Autodesk Inventor part; units mm, degrees
ref_plane "YZ Plane" through (0, 0, 0) normal (1, 0, 0) x (0, 1, 0)
ref_plane "XZ Plane" through (0, 0, 0) normal (0, 1, 0) x (-1, 0, 0)
ref_plane "XY Plane" through (0, 0, 0) normal (0, 0, 1) x (1, 0, 0)
sketch "Skizze1" plane through (0, 0, 0) normal (0, 1, 0) x (-1, 0, 0)
  circle A0 centre (0, 0) radius 12.25
  dimension "d0" = 24.5
extrude "Extrusion1" add sketch "Skizze1" along normal blind 9.5
sketch "Skizze2" plane through (0, 9.5, 0) normal (0, 1, 0) x (1, 0, 0)
  circle A0 centre (0, 0) radius 12.75
  dimension "d3" = 25.5
extrude "Extrusion2" add sketch "Skizze2" along normal blind 1.5
sketch "Skizze3" plane through (0, 0, 0) normal (0, -1, 0) x (1, 0, 0)
  circle A0 centre (0, 0) radius 12.25
hole "Bohrung1" at (0, 0, 0) direction (0, 1, 0) diameter 21 depth 9.5
properties part number "17"
Geometry: final body of the model. Coordinates: model frame, mm. Round coordinates to 2 decimals unless told otherwise and drop trailing zeros. Order: outer loops, then holes, each group sorted by start corner. A loop starts at its lowest first (then second) coordinate and runs counter-clockwise, first axis right, second up. Notation, with made-up numbers: (-13.5, 74) -> (27.5, 74) arc R24 ccw to (27.5, 94) -> close; hole circle Ø9 at (26, 81). An arc over 180 degrees is marked (long way). Put each result on its own line as item: value. Start each with the question number.
Q1. Section A-A on x = 0. Return the cut outline in (y, z).
Q2. Pull-direction query (Z, two-part tool) for faces 1 (the flat face through (0, 9.5, 0)), 2 (the cylindrical face through (-6.586, 4.684, -10.329)), 3 (the cylindrical face through (-3.2, 4.8, -10)), 4 (the flat face through (0, 11, 0)); classes: +Z half, -Z half, draft (parallel to the pull), parting line (faces both ways), or undercut.
Q3. Section D-D on z = 11.25. Return the cut outline in (x, y), and give its area (3 significant figures).
Q4. First-contact query: pin 1 (1 mm diameter, centred on x = 8, y = 4, fed in from -Z); pin 2 (6 mm diameter, centred on y = 9, z = 8.5, fed in from +X); pin 3 (1.5 mm diameter, centred on x = -8.5, z = -3, fed in from -Y). Flat tips, straight axial feed; report the tip coordinate or a pass-through.
Q5. Line query: probe 1 along Z at (x, y) = (0, 5); probe 2 along Y at (x, z) = (4.5, 4.75); probe 3 along X at (y, z) = (6.75, -8.75). Output: solid intervals per line, ascending.
Q6. Section C-C on y = 3. Return the cut outline in (x, z).
Q7. Section B-B on z = 0. Return the cut outline in (x, y).
Ans:
1. outline: (0, -12.25) -> (9.5, -12.25) -> (9.5, -12.75) -> (11, -12.75) -> (11, 12.75) -> (9.5, 12.75) -> (9.5, 12.25) -> (0, 12.25) -> (0, 10.5) -> (9.5, 10.5) -> (9.5, -10.5) -> (0, -10.5) -> close
2. face 1: undercut
2. face 2: parting line
2. face 3: undercut
2. face 4: draft
3. outline: (-6, 9.5) -> (-4.85, 9.5) -> (-4.85, 0) -> (4.85, 0) -> (4.85, 9.5) -> (6, 9.5) -> (6, 11) -> (-6, 11) -> close
3. area: 110 mm2
4. pin 1: stops at z = -9.69
4. pin 2: stops at x = 11.48
4. pin 3: stops at y = 9.5
5. probe 1: z = -12.25 to -10.5, 10.5 to 12.25
5. probe 2: y = 9.5 to 11
5. probe 3: x = -8.57 to -5.8, 5.8 to 8.57
6. outline: circle Ø24.5 at (0, 0); hole circle Ø21 at (0, 0)
7. outline: (-12.75, 9.5) -> (-12.25, 9.5) -> (-12.25, 0) -> (-10.5, 0) -> (-10.5, 9.5) -> (10.5, 9.5) -> (10.5, 0) -> (12.25, 0) -> (12.25, 9.5) -> (12.75, 9.5) -> (12.75, 11) -> (-12.75, 11) -> close
